```python
from build123d import *

# Parameters (mm, degrees)
F0_W     = 1.5
F0_H     = 1.5
F0_W_2   = 19.1
F0_H_2   = 3.5
F0_H_3   = 22.3
F0_H_4   = 5
F0_H_5   = 3
F0_W_3   = 8.857275
F1_DEPTH = 18.1
F2_R     = 1.525
F3_DEPTH = 25


with BuildPart() as f1:
    # F0 (on Top) → F1 (new body)
    with BuildSketch(Plane.XY):
        with Locations((-21.35, 18.05)):
            Rectangle(F0_W, F0_H)
        with Locations((-11.05, 18.05)):
            Rectangle(F0_W_2, F0_H)
        with Locations((-21.35, 15.55)):
            Rectangle(F0_W, F0_H_2)
        with Locations((-0.75, 18.05)):
            Rectangle(F0_W, F0_H)
        with Locations((-0.75, 6.15)):
            Rectangle(F0_W, F0_H_3)
        with Locations((-0.75, -5.75)):
            Rectangle(F0_W, F0_H)
        with Locations((-11.05, -5.75)):
            Rectangle(F0_W_2, F0_H)
        with Locations((-21.35, -5.75)):
            Rectangle(F0_W, F0_H)
        with Locations((-21.35, -2.5)):
            Rectangle(F0_W, F0_H_4)
        with Locations((-21.35, -8)):
            Rectangle(F0_W, F0_H_5)
        with Locations((-16.171363, -10.25)):
            Rectangle(F0_W_3, F0_H)
        with Locations((-21.35, -10.25)):
            Rectangle(F0_W, F0_H)
    extrude(amount=F1_DEPTH)

    # F2 (on face) → F3 (cut)
    with BuildSketch(Plane.YZ):
        with Locations((-2.9, 14.645781)):
            Circle(F2_R)
        with Locations((15.2, 14.645781)):
            Circle(F2_R)
    extrude(amount=-F3_DEPTH, mode=Mode.SUBTRACT)


solid = f1.part
```
Work out the finished part from the listing and answer in its coordinate system (mm). A direction names the side the tool comes from. Round coordinates to 2 decimals unless told otherwise and drop trailing zeros. Write each loop counter-clockwise with the first axis right and the second up, starting at its lowest first coordinate (ties: lowest second). Pieces come first, ordered by that corner, then holes.
1) Which of the six approach directions +Z, -Z, +X, -X, +Y, -Y give full straight-line access (tool end or side, diameter ignored) to faces 5 (the face through (-21, 0, 9)), 6 (the face through (-16, -9.5, 9)), 7 (the face through (-11, -5, 9))?
2) A cutting plane is placed at D-D on y = 3. Determine the outline of the cut face in (x, z).
3) Flat-ended cylindrical pins translate along their axes: P1, Ø4, axis at x = -7, z = 14.5, coming from the -Y side; P2, Ø5, axis at y = -2.9, z = 14.65, coming from the -X side; P3, Ø5.5, axis at y = 3, z = 7.5, coming from the -X side; P4, Ø0.9, axis at y = -8.5, z = 12.5, coming from the +X side. Find the tip coordinate at first contact, or state that the pin passes through.
4) A cutting plane is placed at A-A on y = 15.2. Determine the outline of the cut face in (x, z), and give its area (4 significant figures).
5) A cutting plane is placed at B-B on x = -12.5. Determine the outline of the cut face in (y, z).
6) Determine the mould class of faces 1 (the face through (-1, 5, 18.1)), 2 (the face through (-1, 5, 0)), 3 (the face through (-11, 17.3, 9)), 4 (the face through (-0.74, 15.001, 16.158)) for opening direction Z: pulls with the +Z half, pulls with the -Z half, needs draft (parallel to the pull), parting line crosses it, or undercut.
7) Consider probe 1 along Y at (x, z) = (-17, 9); probe 2 along Y at (x, z) = (-5.5, 4.5); probe 3 along Z at (x, y) = (-0.8, 15.2). Determine where each line is inside the solid, lowest interval first.
8) A cutting plane is placed at C-C on z = 12.5. Determine the outline of the cut face in (x, y).
Entries:
1. face 5: +Z, -Z, -X
1. face 6: +Z, -Z, +X
1. face 7: +Z, -Z
2. outline: (-1.5, 0) - (0, 0) - (0, 18.1) - (-1.5, 18.1) - close
3. P1: stops at y = -6.5
3. P2: stops at x = -22.1
3. P3: stops at x = -1.5
3. P4: stops at x = -20.6
4. outline: (-22.1, 0) - (-20.6, 0) - (-20.6, 13.12) - (-22.1, 13.12) - close; (-22.1, 16.17) - (-20.6, 16.17) - (-20.6, 18.1) - (-22.1, 18.1) - close; (-1.5, 0) - (0, 0) - (0, 13.12) - (-1.5, 13.12) - close; (-1.5, 16.17) - (0, 16.17) - (0, 18.1) - (-1.5, 18.1) - close
4. area: 45.15 mm2
5. outline: (-11, 0) - (-9.5, 0) - (-9.5, 18.1) - (-11, 18.1) - close; (-6.5, 0) - (-5, 0) - (-5, 18.1) - (-6.5, 18.1) - close; (17.3, 0) - (18.8, 0) - (18.8, 18.1) - (17.3, 18.1) - close
6. face 1: pulls with the +Z half
6. face 2: pulls with the -Z half
6. face 3: needs draft
6. face 4: undercut
7. probe 1: y = -11 to -9.5, -6.5 to -5, 17.3 to 18.8
7. probe 2: y = -6.5 to -5, 17.3 to 18.8
7. probe 3: z = 0 to 13.12, 16.17 to 18.1
8. outline: (-22.1, -11) - (-11.74, -11) - (-11.74, -9.5) - (-20.6, -9.5) - (-20.6, -6.5) - (0, -6.5) - (0, 18.8) - (-22.1, 18.8) - (-22.1, 13.8) - (-20.6, 13.8) - (-20.6, 17.3) - (-1.5, 17.3) - (-1.5, -5) - (-20.6, -5) - (-20.6, 0) - (-22.1, 0) - close
